Here's the drawing with two shaded views (mm, measured from the low corner). I have some questions. A direction names the side the tool comes from. Round coordinates to 2 decimals unless told otherwise and drop trailing zeros. Loops run counter-clockwise (first coordinate to the right, second up) from the corner with the lowest first, then second, coordinate; pieces in that order, holes last. Notation, with made-up numbers: (71.5, 6) -> (104.5, 6) arc R20 ccw to (104.5, 35) -> close; hole circle Ø6 at (78, -4). An arc over 180 degrees is marked (long way). One line per item, written item: value. Start each with the question number.
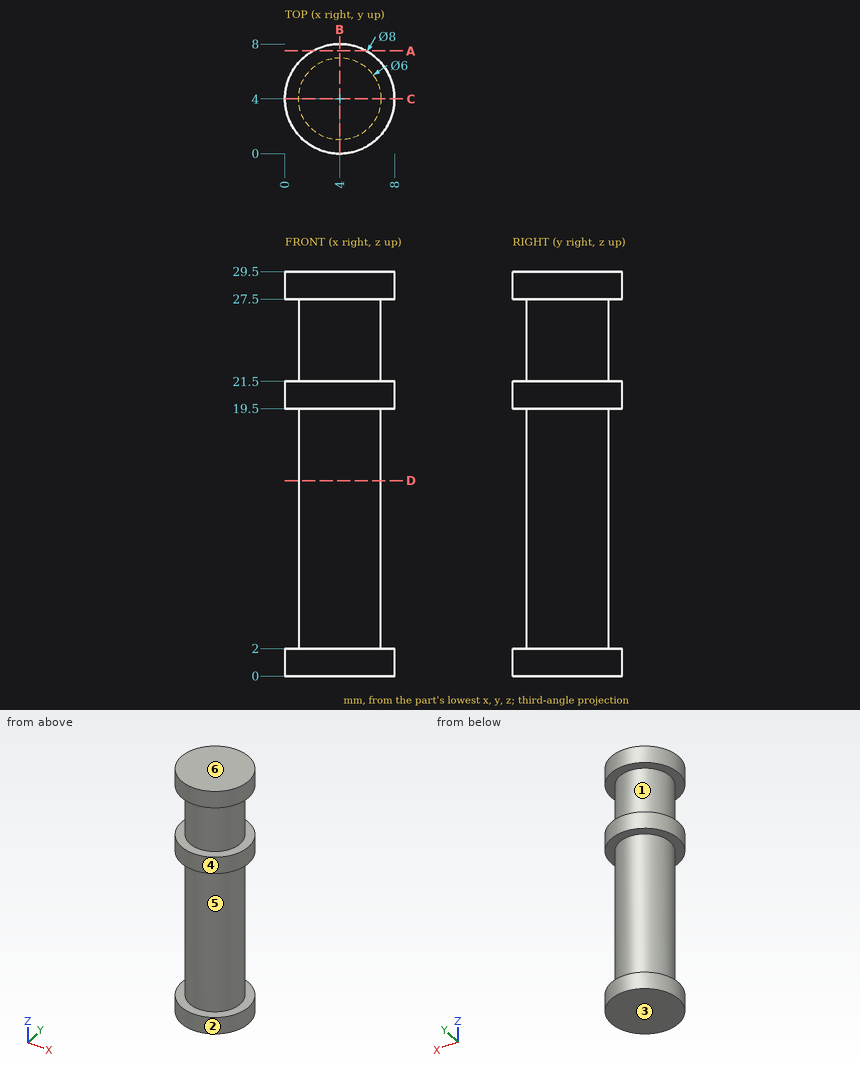
Q1. I want a section at B-B on x = 4. Please give me the cut outline in (y, z).
Q2. Will this pin go through, and if not, where does the flat tip stop? P1, Ø1.5, axis at x = 5, z = 15.5, coming from the +Y side.
Q3. I want a section at A-A on y = 7.5. Please give me the cut outline in (x, z), plus the area to 3 significant figures.
Q4. If I drill on line 1 along Z through (x, y) = (0.5, 2.25); line 2 along X through (y, z) = (4, 26.5); line 3 along Y through (x, z) = (5.75, 4), over which ranges is the centre line in solid material (lowest first)?
Q5. Which directions (+Z, -Z, +X, -X, +Y, -Y) give clear straight access to the entire face, cutting with the end or side of a thin tool? Please do the marked faces 1 and 2.
Q6. If we mould it in two halves opening along Z, with no side actions, what happens to the marked faces 3, 4, 5 and 6? For each: released by +Z, released by -Z, zero draft, split by the parting line, or undercut.
Q7. I want a section at D-D on z = 14.25. Please give me the cut outline in (x, y).
Answers below:
1. outline: (0, 0) -> (8, 0) -> (8, 2) -> (7, 2) -> (7, 19.5) -> (8, 19.5) -> (8, 21.5) -> (7, 21.5) -> (7, 27.5) -> (8, 27.5) -> (8, 29.5) -> (0, 29.5) -> (0, 27.5) -> (1, 27.5) -> (1, 21.5) -> (0, 21.5) -> (0, 19.5) -> (1, 19.5) -> (1, 2) -> (0, 2) -> close
2. P1: stops at y = 6.99
3. outline: (2.06, 0) -> (5.94, 0) -> (5.94, 2) -> (2.06, 2) -> close; (2.06, 19.5) -> (5.94, 19.5) -> (5.94, 21.5) -> (2.06, 21.5) -> close; (2.06, 27.5) -> (5.94, 27.5) -> (5.94, 29.5) -> (2.06, 29.5) -> close
3. area: 23.2 mm^2
4. line 1: z = 0 to 2, 19.5 to 21.5, 27.5 to 29.5
4. line 2: x = 1 to 7
4. line 3: y = 1.56 to 6.44
5. face 1: none
5. face 2: +Z, -Z
6. face 3: released by -Z
6. face 4: zero draft
6. face 5: undercut
6. face 6: released by +Z
7. outline: circle Ø6 at (4, 4)
